Source: CAD feature listing. Evaluate the final solid. Frame: model axes, mm. A direction names the side the tool comes from. Give positions to 0.01 mm unless a question says otherwise; leave off trailing zeros. Order: outer loops, then holes, each group sorted by start corner. A loop starts at its lowest first (then second) coordinate and runs counter-clockwise, first axis right, second up. Notation, with made-up numbers: (-26.5, 79) - (-8.5, 79) arc R24 ccw to (-8.5, 114) - close; hole circle Ø6 at (71.25, 78). An arc over 180 degrees is marked (long way). Write each question's results on one line, items separated by ' | '. Start each with the question number.
Item 1: Line query: line 1 along Y through (x, z) = (19, 33); line 2 along Z through (x, y) = (-29.5, -24); line 3 along X through (y, z) = (-6.5, 30). Output: solid intervals per line, ascending.
Item 2: Set-up query: faces 5 (the flat face through (-1, -25.5, -6)), 6 (the cylindrical face through (24.54, -8.8, 31.42)). Return all of +Z, -Z, +X, -X, +Y, -Y with unobstructed straight access to the full face (end or side cutting, diameter ignored); none if empty.
Item 3: Contact query for a flat-ended pin moving along its axis: pin 1 Ø6 at (x, z) = (0, 0) entering from -Y. Output: stop coordinate, or through.
Item 4: Section B-B on x = 0. Output: boundary loops of the cut face in (y, z), and give its area (3 significant figures).
Item 5: Section D-D on y = -6.5. Output: boundary loops of the cut face in (x, z).
Item 6: Section C-C on x = 19. Output: boundary loops of the cut face in (y, z).
Item 7: Section A-A on z = 0. Output: boundary loops of the cut face in (x, y).
Item 8: Mould query, pull axis X, two halves, no side actions, for faces 1 (the cylindrical face through (-23.76, -10.15, 31.42)), 2 (the flat face through (-1, -37.5, 9)), 3 (the cylindrical face through (-46.288, -12.112, 31.584)), 4 (the flat face through (72, -32, 1)). Classes: released by +X, released by -X, zero draft, split by the parting line, or undercut.
```python
from build123d import *

# Parameters (mm, degrees)
SKETCH1_R           = 6
SKETCH1_W           = 72
SKETCH1_H           = 12
BOSS_EXTRUDE1_DEPTH = 37.5
SKETCH2_W           = 164.389356844
SKETCH2_H           = 51
CUT_EXTRUDE1_DEPTH  = 38
SKETCH3_R           = 5
CUT_EXTRUDE2_DEPTH  = 90.633977932


with BuildPart() as part:
    # Sketch1 → Boss-Extrude1 (new, symmetric)
    # profile 1 of 4: a face of its own
    with BuildSketch(Plane.XY):
        with BuildLine():
            ThreePointArc((-32.5, 12.5), (-46.579087682, -12.39476412), (-72, -25.5))
            Line((-72, -25.5), (0, -25.5))
            Line((0, -25.5), (0, 12.5))
            Line((0, 12.5), (-32.5, 12.5))
        make_face()
        with Locations((-19, -6.5)):
            Circle(SKETCH1_R, mode=Mode.SUBTRACT)
    # profile 2 of 4: a face of its own
    with BuildSketch(Plane.XY):
        with BuildLine():
            Line((0, 12.5), (0, -25.5))
            Line((0, -25.5), (72, -25.5))
            ThreePointArc((72, -25.5), (46.579087682, -12.39476412), (32.5, 12.5))
            Line((32.5, 12.5), (0, 12.5))
        make_face()
        with Locations((19, -6.5)):
            Circle(SKETCH1_R, mode=Mode.SUBTRACT)
    # profile 3 of 4: a face of its own
    with BuildSketch(Plane.XY):
        with Locations((-36, -31.5)):
            Rectangle(SKETCH1_W, SKETCH1_H)
    # profile 4 of 4: a face of its own
    with BuildSketch(Plane.XY):
        with Locations((36, -31.5)):
            Rectangle(SKETCH1_W, SKETCH1_H)
    extrude(amount=BOSS_EXTRUDE1_DEPTH, both=True)

    # Sketch2 → Cut-Extrude1 (cut)
    with BuildSketch(Plane(origin=(0, 12.5, 0), x_dir=(1, 0, 0), z_dir=(0, 1, 0))):
        Rectangle(SKETCH2_W, SKETCH2_H)
    extrude(amount=-CUT_EXTRUDE1_DEPTH, mode=Mode.SUBTRACT)

    # Sketch3 → Cut-Extrude2 (cut, through all)
    with BuildSketch(Plane(origin=(0, -25.5, 0), x_dir=(1, 0, 0), z_dir=(0, 1, 0))):
        with Locations(Location((0, 0, 0), (0, 0, 180))):
            Circle(SKETCH3_R)
    extrude(amount=-CUT_EXTRUDE2_DEPTH, mode=Mode.SUBTRACT)


solid = part.part
```
Evaluation:
1) line 1: y = -37.5 to -12.5, -0.5 to 12.5 | line 2: z = -37.5 to -25.5, 25.5 to 37.5 | line 3: x = -41.35 to -25, -13 to 13, 25 to 41.35
2) face 5: +X, -X, +Y | face 6: +Z, -Z
3) pin 1: passes through
4) outline: (-37.5, -37.5) - (12.5, -37.5) - (12.5, -25.5) - (-25.5, -25.5) - (-25.5, -5) - (-37.5, -5) - close; (-37.5, 5) - (-25.5, 5) - (-25.5, 25.5) - (12.5, 25.5) - (12.5, 37.5) - (-37.5, 37.5) - close | area: 1,690 mm^2
5) outline: (-41.35, -37.5) - (-25, -37.5) - (-25, -25.5) - (-41.35, -25.5) - close; (-41.35, 25.5) - (-25, 25.5) - (-25, 37.5) - (-41.35, 37.5) - close; (-13, -37.5) - (13, -37.5) - (13, -25.5) - (-13, -25.5) - close; (-13, 25.5) - (13, 25.5) - (13, 37.5) - (-13, 37.5) - close; (25, -37.5) - (41.35, -37.5) - (41.35, -25.5) - (25, -25.5) - close; (25, 25.5) - (41.35, 25.5) - (41.35, 37.5) - (25, 37.5) - close
6) outline: (-37.5, -37.5) - (-12.5, -37.5) - (-12.5, -25.5) - (-25.5, -25.5) - (-25.5, 25.5) - (-12.5, 25.5) - (-12.5, 37.5) - (-37.5, 37.5) - close; (-0.5, -37.5) - (12.5, -37.5) - (12.5, -25.5) - (-0.5, -25.5) - close; (-0.5, 25.5) - (12.5, 25.5) - (12.5, 37.5) - (-0.5, 37.5) - close
7) outline: (-72, -37.5) - (-5, -37.5) - (-5, -25.5) - (-72, -25.5) - close; (5, -37.5) - (72, -37.5) - (72, -25.5) - (5, -25.5) - close
8) face 1: undercut | face 2: zero draft | face 3: released by -X | face 4: released by +X
